from build123d import *

# Parameters (mm, degrees)
EXTRUDE_1_DEPTH     = 10
CUT_EXTRUDE_1_REACH = 106.47
SKETCH_2_R          = 4


# Read off the part's stored shape, not the designer's step: 高级异型孔1
with BuildPart() as part:
    # 草图1 → 凸台-拉伸1 (new body)
    with BuildSketch(Plane.XY.offset(58)):
        with BuildLine():
            Line((31, 26), (18, 26))
            Line((18, 26), (18, 31))
            Line((18, 31), (33.354781752, 44.199646864))
            ThreePointArc((33.354781752, 44.199646864), (56.673182808, 48.74032246), (72.473389189, 31))
            Line((72.473389189, 31), (77, 31))
            Line((77, 31), (77, 26))
            Line((77, 26), (67, 26))
            ThreePointArc((67, 26), (49, 44), (31, 26))
        make_face()
    extrude(amount=EXTRUDE_1_DEPTH)

    # 草图2 → 切除-拉伸1 (cut, up to next)
    with BuildSketch(Plane(origin=(0, 31, 0), x_dir=(1, 0, 0), z_dir=(0, 1, 0)), mode=Mode.PRIVATE) as cut_extrude_1_sk1:
        with Locations(Location((26, -63, 0), (0, 0, 180))):
            Circle(SKETCH_2_R)
    cut_extrude_1_tool1 = extrude(cut_extrude_1_sk1.sketch, amount=CUT_EXTRUDE_1_REACH, mode=Mode.PRIVATE) & part.part
    # 草图2 → 切除-拉伸1 (cut, up to next)
    with BuildSketch(Plane(origin=(0, 31, 0), x_dir=(1, 0, 0), z_dir=(0, 1, 0)), mode=Mode.PRIVATE) as cut_extrude_1_sk2:
        with Locations((72, -63)):
            Circle(SKETCH_2_R)
    cut_extrude_1_tool2 = extrude(cut_extrude_1_sk2.sketch, amount=CUT_EXTRUDE_1_REACH, mode=Mode.PRIVATE) & part.part
    add(cut_extrude_1_tool1.solids().sort_by_distance((26, 31, 63))[0], mode=Mode.SUBTRACT)
    add(cut_extrude_1_tool2.solids().sort_by_distance((72, 31, 63))[0], mode=Mode.SUBTRACT)

    # 高级异型孔1 outline → 高级异型孔1 (revolve, cut)
    with BuildSketch(Plane(origin=(72, 0, 63), x_dir=(1, 0, 0), z_dir=(0, 0, 1))):
        Polygon((0, 26), (2.25, 26), (2.25, 28.55), (4.7, 31), (0, 31), align=None)
    revolve(axis=Axis((72, 0, 63), (0, 1, 0)), mode=Mode.SUBTRACT)

    # Other 1 2 outline → Other 1 2 (revolve, cut)
    with BuildSketch(Plane(origin=(26, 0, 63), x_dir=(1, 0, 0), z_dir=(0, 0, 1))):
        Polygon((4.7, 31), (0, 31), (0, 26), (2.25, 26), (2.25, 28.55), align=None)
    revolve(axis=Axis((26, 0, 63), (0, 1, 0)), mode=Mode.SUBTRACT)


solid = part.part
Input: part model. Units: mm. Frame: model coordinates. A direction names the side the tool comes from. Round coordinates to 2 decimals unless told otherwise and drop trailing zeros. Order: outer loops, then holes, each group sorted by start corner. A loop starts at its lowest first (then second) coordinate and runs counter-clockwise, first axis right, second up. Notation, with made-up numbers: (15.5, 65.25) - (49.5, 65.25) arc R28 cw to (49.5, 90.25) - close; hole circle Ø4 at (18.5, -6.75). An arc over 180 degrees is marked (long way). Use a Markdown table: item, result.
1. Material intervals for probe 1 along Z at (x, y) = (26, 27.6); probe 2 along X at (y, z) = (26.6, 63); probe 3 along X at (y, z) = (28, 63), sorted ascending.
Evaluation:
| item | result |
|---|---|
| probe 1 | 58 to 60.75, 65.25 to 68 |
| probe 2 | 18 to 23.75, 28.25 to 31.01, 66.99 to 69.75, 74.25 to 77 |
| probe 3 | 18 to 23.75, 28.25 to 31.11, 66.89 to 69.75, 74.25 to 77 |
2. Mould query, pull axis Y, two halves, no side actions, for faces 4 (the face through (49, 44, 63)), 5 (the face through (77, 29, 63)), 6 (the face through (67.8, 31, 62.6)), 7 (the face through (28, 31, 59)). Classes: +Y half, -Y half, draft (parallel to the pull), parting line (faces both ways), or undercut.
Evaluation:
| item | result |
|---|---|
| face 4 | -Y half |
| face 5 | draft |
| face 6 | undercut |
| face 7 | undercut |
3. First-contact query: pin 1 (2.5 mm diameter, centred on x = 72, z = 63, fed in from +Y); pin 2 (5 mm diameter, centred on x = 26, z = 63, fed in from -Y); pin 3 (5 mm diameter, centred on x = 55, z = 66, fed in from -Y); pin 4 (3 mm diameter, centred on y = 42, z = 63, fed in from +X). Flat tips, straight axial feed; report the tip coordinate or a pass-through.
Evaluation:
| item | result |
|---|---|
| pin 1 | through |
| pin 2 | y = 26 |
| pin 3 | y = 41.87 |
| pin 4 | x = 68.04 |
4. Section C-C on z = 63. Return the cut outline in (x, y), then the cut area to 3 significant figures.
Evaluation:
| item | result |
|---|---|
| outline | (18, 26) - (23.75, 26) - (23.75, 28.55) - (21.3, 31) - (22, 31) - (22, 34.44) - (18, 31) - close; (28.25, 26) - (31, 26) arc R18 cw to (67, 26) - (69.75, 26) - (69.75, 28.55) - (67.3, 31) - (68, 31) - (68, 40.66) arc R24 ccw to (33.35, 44.2) - (30, 41.32) - (30, 31) - (30.7, 31) - (28.25, 28.55) - close; (74.25, 26) - (77, 26) - (77, 31) - (76.7, 31) - (74.25, 28.55) - close |
| area | 351 mm^2 |
5. Section D-D on y = 36.75. Return the cut outline in (x, z).
Evaluation:
| item | result |
|---|---|
| outline | (24.69, 58) - (34.56, 58) - (34.56, 68) - (24.69, 68) - (24.69, 66.78) arc R4 cw (long way) to (24.69, 59.22) - close; (63.44, 58) - (70.46, 58) - (70.46, 59.31) arc R4 cw to (70.46, 66.69) - (70.46, 68) - (63.44, 68) - close |
6. Access query for faces 1 (the face through (76.74, 31, 64.09)), 2 (the face through (27.11, 28.7, 65.13)), 3 (the face through (30, 35, 63)). Directions: +Z, -Z, +X, -X, +Y, -Y. A direction counts if a zero-diameter tool reaches every point of the face in a straight line with its end or side. Return the directions, or none.
Evaluation:
| item | result |
|---|---|
| face 1 | +Z, -Z, +X, +Y |
| face 2 | none |
| face 3 | +Y |
7. Section A-A on x = 26. Return the cut outline in (y, z).
Evaluation:
| item | result |
|---|---|
| outline | (26, 58) - (37.88, 58) - (37.88, 59) - (31, 59) - (31, 58.3) - (28.55, 60.75) - (26, 60.75) - close; (26, 65.25) - (28.55, 65.25) - (31, 67.7) - (31, 67) - (37.88, 67) - (37.88, 68) - (26, 68) - close |
8. Section B-B on y = 33.75. Return the cut outline in (x, z).
Evaluation:
| item | result |
|---|---|
| outline | (21.2, 58) - (32.75, 58) - (32.75, 68) - (21.2, 68) - close; (65.25, 58) - (71.71, 58) - (71.71, 59.01) arc R4 cw to (71.71, 66.99) - (71.71, 68) - (65.25, 68) - close; hole circle Ø8 at (26, 63) |
